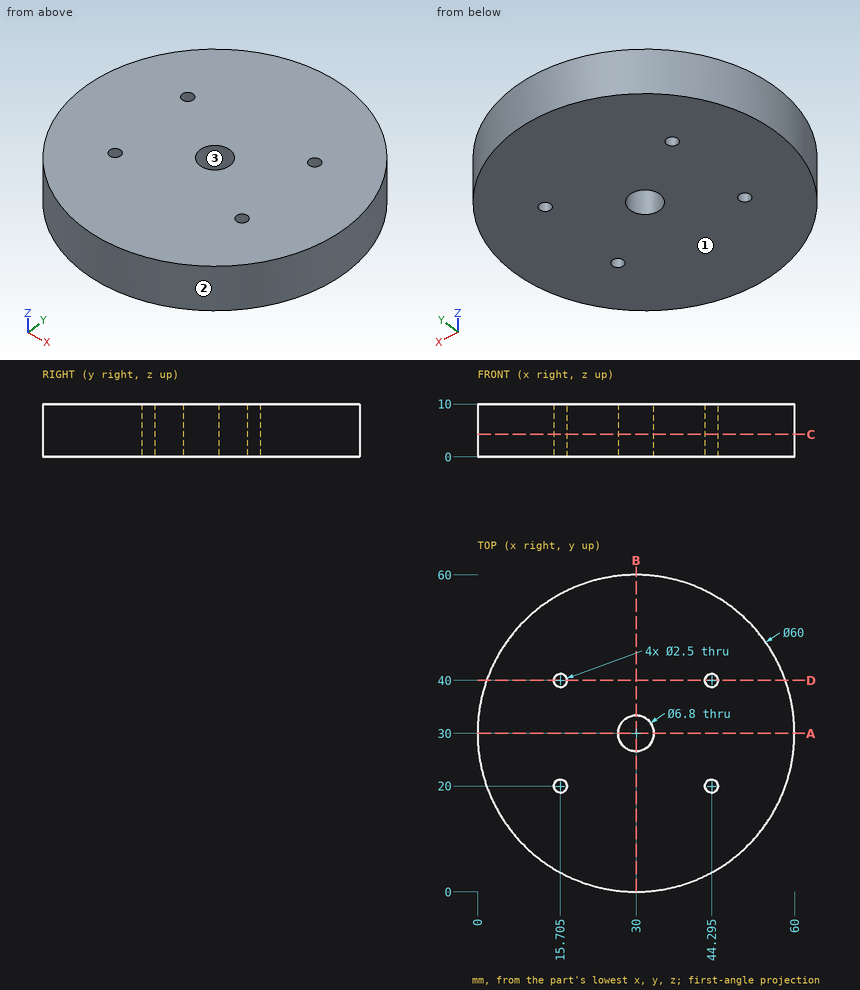
Input: dimensioned drawing with shaded views. Units: mm. Origin: part minimum x, y, z. Round coordinates to 2 decimals unless told otherwise and drop trailing zeros. Order: outer loops, then holes, each group sorted by start corner. A loop starts at its lowest first (then second) coordinate and runs counter-clockwise, first axis right, second up.
Q1. Section C-C, the plane z = 4.25. Output: boundary loops of the cut face in (x, y) (3 decimals), and give its area (3 significant figures).
Result sheet:
outline: circle Ø60 at (30, 30); hole circle Ø2.5 at (15.705, 20); hole circle Ø2.5 at (15.705, 40); hole circle Ø6.8 at (30, 30); hole circle Ø2.5 at (44.295, 20); hole circle Ø2.5 at (44.295, 40)
area: 2,770 mm2
Q2. Material intervals for probe 1 along X at (y, z) = (20, 5) (3 decimals); probe 2 along X at (y, z) = (30.5, 4); probe 3 along Y at (x, z) = (30, 5), sorted ascending.
Result sheet:
probe 1: x = 1.716 to 14.455, 16.955 to 43.045, 45.545 to 58.284
probe 2: x = 0 to 26.64, 33.36 to 60
probe 3: y = 0 to 26.6, 33.4 to 60
Q3. Mould query, pull axis X, two halves, no side actions, for the marked faces 1, 2 and 3. Classes: released by +X, released by -X, zero draft, split by the parting line, or undercut.
Result sheet:
face 1: zero draft
face 2: split by the parting line
face 3: undercut
Q4. Section A-A, the plane y = 30. Output: boundary loops of the cut face in (x, z), and give its area (3 significant figures).
Result sheet:
outline: (0, 0) - (26.6, 0) - (26.6, 10) - (0, 10) - close; (33.4, 0) - (60, 0) - (60, 10) - (33.4, 10) - close
area: 532 mm2
Q5. Section D-D, the plane y = 40. Output: boundary loops of the cut face in (x, z) (3 decimals).
Result sheet:
outline: (1.716, 0) - (14.455, 0) - (14.455, 10) - (1.716, 10) - close; (16.955, 0) - (43.045, 0) - (43.045, 10) - (16.955, 10) - close; (45.545, 0) - (58.284, 0) - (58.284, 10) - (45.545, 10) - close
Q6. Pin query (flat end, axial travel): pin 1 (4 mm diameter, centred on x = 17, z = 8, fed in from +Y); pin 2 (1.5 mm diameter, centred on x = 44.295, y = 20, fed in from +Z); pin 3 (1 mm diameter, centred on x = 28, z = 7, fed in from -Y). Return the tip coordinate at first contact, or that it passes through.
Result sheet:
pin 1: stops at y = 57.91
pin 2: passes through
pin 3: stops at y = 0.04
